Source: CAD feature listing. Evaluate the final solid. Frame: model axes, mm. A direction names the side the tool comes from. Round coordinates to 2 decimals unless told otherwise and drop trailing zeros. Order: outer loops, then holes, each group sorted by start corner. A loop starts at its lowest first (then second) coordinate and runs counter-clockwise, first axis right, second up. Notation, with made-up numbers: M 34,-10.75 L 73,-10.75 A23 cw 73,22.25 Z; hole C 26,51 d7. An arc over 180 degrees is marked long. Use one line per item in the form item = value. Start each with the question number.
Q1. Reachability of faces 5 (the flat face through (-2, 65, 9.6)), 6 (the flat face through (56.243, 49, 4)) from +Z, -Z, +X, -X, +Y, -Y: full face, straight path, thin tool, end or side. Return the list, or none.
Q2. Section A-A (x = 40.5). Return the cut outline in (y, z), plus the area to 3 significant figures.
Q3. Material intervals for probe 1 along Y at (x, z) = (8, 5.5); probe 2 along X at (y, z) = (67, 4.5); probe 3 along X at (y, z) = (33, 1.25), sorted ascending.
Q4. Section B-B (z = 6.5). Return the cut outline in (x, y).
Q5. Contact query for flat-ended pins moving along their axis: pin 1 (2.5 mm diameter, centred on x = -8.76, y = 33.41, fed in from +Z); pin 2 (1.5 mm diameter, centred on x = 19, y = 45.5, fed in from +Z); pin 3 (0.8 mm diameter, centred on x = -13, y = 46.5, fed in from +Z). Output: stop coordinate, or through.
Q6. Section C-C (y = 59.5). Return the cut outline in (x, z), plus the area to 4 significant figures.
Q7. Pull-direction query (Y, two-part tool) for faces 1 (the flat face through (22, 69.411, 4)), 2 (the flat face through (21, 49, 0)), 3 (the flat face through (21, 28.411, 4)), 4 (the cylindrical face through (46.173, 65.362, 5.493)); classes: pulls with the +Y half, pulls with the -Y half, needs draft (parallel to the pull), parting line crosses it, or undercut.
from build123d import *

# Parameters (mm, degrees)
F0_R           = 2
F0_R_2         = 1.5
F0_W           = 1
F0_H           = 20
F1_DEPTH       = 1.5
F2_DEPTH       = 7.5
F3_DEPTH       = 9.6
F4_DEPTH       = 3.5
F5_D           = 3
F5_CSINK_D     = 5.5
F5_CSINK_ANGLE = 90


with BuildPart() as f1:
    # F0 (on Top) → F1 (new body)
    with BuildSketch(Plane.XY):
        Polygon((56.2425711751, 68.4110085815), (-12.7574288249, 68.4110085815), (-12.7574288249, 57.4110085815), (-12.7574288249, 37.4110085815), (-12.7574288249, 29.4110085815), (56.2425711751, 29.4110085815), align=None)
        with Locations((-8.7574288249, 33.4110085815)):
            Circle(F0_R, mode=Mode.SUBTRACT)
        with Locations((-2.2574288249, 33.9110085815)):
            Circle(F0_R_2, mode=Mode.SUBTRACT)
        with Locations((52.2425711751, 33.4110085815)):
            Circle(F0_R, mode=Mode.SUBTRACT)
        with Locations((44.7425711751, 33.9110085815)):
            Circle(F0_R_2, mode=Mode.SUBTRACT)
        with Locations((-8.7574288249, 64.4110085815)):
            Circle(F0_R, mode=Mode.SUBTRACT)
        with Locations((-1.8220887287, 64.9110085815)):
            Circle(F0_R_2, mode=Mode.SUBTRACT)
        with Locations((44.7425711751, 64.9110085815)):
            Circle(F0_R_2, mode=Mode.SUBTRACT)
        with Locations((52.2425711751, 64.4110085815)):
            Circle(F0_R, mode=Mode.SUBTRACT)
        Polygon((-12.7574288249, 57.4110085815), (-12.7574288249, 68.4110085815), (56.2425711751, 68.4110085815), (56.2425711751, 29.4110085815), (-12.7574288249, 29.4110085815), (-12.7574288249, 37.4110085815), (-13.7574288249, 37.4110085815), (-13.7574288249, 28.4110085815), (57.2425711751, 28.4110085815), (57.2425711751, 69.4110085815), (-13.7574288249, 69.4110085815), (-13.7574288249, 57.4110085815), align=None)
        with Locations((-2.2574288249, 33.9110085815)):
            Circle(F0_R_2)
        with Locations((44.7425711751, 33.9110085815)):
            Circle(F0_R_2)
        with Locations((44.7425711751, 64.9110085815)):
            Circle(F0_R_2)
        with Locations((-1.8220887287, 64.9110085815)):
            Circle(F0_R_2)
        with Locations((-13.2574288249, 47.4110085815)):
            Rectangle(F0_W, F0_H)
    extrude(amount=F1_DEPTH)

    # F0 (on Top) → F2 (join)
    with BuildSketch(Plane.XY):
        Polygon((-12.7574288249, 57.4110085815), (-12.7574288249, 68.4110085815), (56.2425711751, 68.4110085815), (56.2425711751, 29.4110085815), (-12.7574288249, 29.4110085815), (-12.7574288249, 37.4110085815), (-13.7574288249, 37.4110085815), (-13.7574288249, 28.4110085815), (57.2425711751, 28.4110085815), (57.2425711751, 69.4110085815), (-13.7574288249, 69.4110085815), (-13.7574288249, 57.4110085815), align=None)
    extrude(amount=F2_DEPTH)

    # F0 (on Top) → F3 (join)
    with BuildSketch(Plane.XY):
        with Locations((-1.8220887287, 64.9110085815)):
            Circle(F0_R_2)
        with Locations((-2.2574288249, 33.9110085815)):
            Circle(F0_R_2)
        with Locations((44.7425711751, 33.9110085815)):
            Circle(F0_R_2)
        with Locations((44.7425711751, 64.9110085815)):
            Circle(F0_R_2)
    extrude(amount=F3_DEPTH)

    # F0 (on Top) → F4 (join)
    with BuildSketch(Plane.XY):
        with Locations((-13.2574288249, 47.4110085815)):
            Rectangle(F0_W, F0_H)
    extrude(amount=F4_DEPTH)

    # F5 (through all)
    with Locations(Plane(origin=(0, 0, 0), x_dir=(1, 0, 0), z_dir=(0, 0, -1))):
        with Locations((52.2425711751, -64.4110085815), (52.2425711751, -33.4110085815), (-8.7574288249, -33.4110085815), (-8.7574288249, -64.4110085815)):
            CounterSinkHole(F5_D / 2, F5_CSINK_D / 2, counter_sink_angle=F5_CSINK_ANGLE)


solid = f1.part
Results list:
q1.face_5 = +Z, +X, -X, +Y, -Y
q1.face_6 = +Z
q2.outline = M 28.41,0 L 69.41,0 L 69.41,7.5 L 68.41,7.5 L 68.41,1.5 L 29.41,1.5 L 29.41,7.5 L 28.41,7.5 Z
q2.area = 73.5 mm2
q3.probe_1 = 28.41 to 29.41, 68.41 to 69.41
q3.probe_2 = -13.76 to -12.76, 56.24 to 57.24
q3.probe_3 = -13.76 to -10.71, -6.8 to 50.29, 54.2 to 57.24
q4.outline = M -13.76,28.41 L 57.24,28.41 L 57.24,69.41 L -13.76,69.41 L -13.76,57.41 L -12.76,57.41 L -12.76,68.41 L 56.24,68.41 L 56.24,29.41 L -12.76,29.41 L -12.76,37.41 L -13.76,37.41 Z; C -2.26,33.91 d3; C -1.82,64.91 d3; C 44.74,33.91 d3; C 44.74,64.91 d3
q5.pin_1 = through
q5.pin_2 = 1.5
q5.pin_3 = 3.5
q6.outline = M -13.76,0 L 57.24,0 L 57.24,7.5 L 56.24,7.5 L 56.24,1.5 L -12.76,1.5 L -12.76,7.5 L -13.76,7.5 Z
q6.area = 118.5 mm2
q7.face_1 = pulls with the +Y half
q7.face_2 = needs draft
q7.face_3 = pulls with the -Y half
q7.face_4 = undercut
